Design review of the part built by this model. Coordinates are the model's own, in mm. A direction names the side the tool comes from. Round coordinates to 2 decimals unless told otherwise and drop trailing zeros. Write each loop counter-clockwise with the first axis right and the second up, starting at its lowest first coordinate (ties: lowest second). Pieces come first, ordered by that corner, then holes. Notation, with made-up numbers: (46, -26.5) - (85, -26.5) arc R9 cw to (85, -20.5) - close; hole circle Ø11 at (19, -24). An arc over 180 degrees is marked (long way). Use one line per item in the form item = value.
```python
from build123d import *

# Parameters (mm, degrees)
F1_DEPTH = 46.6
F2_W     = 38.3587293327
F2_H     = 9.7292885184
F3_DEPTH = 83.7873460183
F6_DEPTH = 23.8091403077


with BuildPart() as f1:
    # F0 (on Right) → F1 (new body, symmetric)
    with BuildSketch(Plane.YZ):
        Polygon((0, 19.4585770369), (0, 0), (83.7863460183, 0), (83.7863460183, 43.2667173445), align=None)
    extrude(amount=F1_DEPTH, both=True)

    # F2 (on face) → F3 (cut, through all)
    with BuildSketch(Plane.XZ):
        with Locations((0, 4.8646442592)):
            Rectangle(F2_W, F2_H)
    extrude(amount=-F3_DEPTH, mode=Mode.SUBTRACT)

    # F5 (on plane+point) → F6 (cut, through all)
    with BuildSketch(Plane.XY.offset(19.4585770369)):
        with BuildLine():
            Line((-19.1793646663, 0), (19.1793646663, 0))
            Line((19.1793646663, 0), (0.097478719, 83.3605036706))
            ThreePointArc((0.097478719, 83.3605036706), (0, 83.4381900123), (-0.097478719, 83.3605036706))
            Line((-0.097478719, 83.3605036706), (-19.1793646663, 0))
        make_face()
    extrude(amount=F6_DEPTH, mode=Mode.SUBTRACT)


solid = f1.part
```
Q1. We need section B-B on y = 35.5. Write out the cut boundary in (x, z), then the cut area to 3 significant figures.
Calculated:
outline = (-46.6, 0) - (-19.18, 0) - (-19.18, 9.73) - (19.18, 9.73) - (19.18, 0) - (46.6, 0) - (46.6, 29.55) - (11.05, 29.55) - (11.05, 19.46) - (-11.05, 19.46) - (-11.05, 29.55) - (-46.6, 29.55) - close
area = 2,160 mm2
Q2. We need section D-D on z = 34.5. Write out the cut boundary in (x, y), then the cut area to 3 significant figures.
Calculated:
outline = (-46.6, 52.93) - (-7.06, 52.93) - (-0.1, 83.36) arc R0.1 cw to (0.1, 83.36) - (7.06, 52.93) - (46.6, 52.93) - (46.6, 83.79) - (-46.6, 83.79) - close
area = 2,660 mm2
Q3. To check wall thickness, follow line 1 along X through (y, z) = (58.5, 2); line 2 along X through (y, z) = (42, 21.5); line 3 along Z through (x, y) = (3, 67). State the ranges of each line that lie inside material, in increasing order. Write a range as from..to.
Calculated:
line_1 = -46.6..-19.18, 19.18..46.6
line_2 = -46.6..-9.57, 9.57..46.6
line_3 = 9.73..19.46
Q4. We need section C-C on x = -2. Write out the cut boundary in (y, z), then the cut area to 3 significant figures.
Calculated:
outline = (0, 9.73) - (83.79, 9.73) - (83.79, 43.27) - (75.05, 40.78) - (75.05, 19.46) - (0, 19.46) - close
area = 1,010 mm2
Q5. Machinability: for faces 4 (the flat face through (33, 41, 0)), 5 (the flat face through (5.53, 59.62, 25.87)), 6 (the flat face through (19.179, 41, 5)), which of the approach directions +Z, -Z, +X, -X, +Y, -Y give a long, thin tool a straight path to every point of the face, cutting with its end or side? Answer none if there is none.
Calculated:
face_4 = -Z, +X, -X, +Y, -Y
face_5 = +Z, -Y
face_6 = -Z, +Y, -Y
Q6. For P1, Ø8, axis at x = 9.5, y = 66, coming from the -Z side; P2, Ø10, axis at x = 18.5, y = 63.5, coming from the +Z side; P3, Ø1.5, axis at x = -4.5, y = 62, coming from the +Z side, all flat-tipped, find the tip position at first contact; note any pin that passes through.
Calculated:
P1 = 9.73
P2 = 38.92
P3 = 37.27
Q7. Draft analysis for pull direction X (two halves, no side actions). For faces 1 (the flat face through (0, 33, 19.459)), 2 (the flat face through (1, 0, 10)), 3 (the flat face through (-46.6, 51, 17)), state which applies: released by +X, released by -X, zero draft, split by the parting line, or undercut.
Calculated:
face_1 = undercut
face_2 = zero draft
face_3 = released by -X
Q8. We need section A-A on z = 4. Write out the cut boundary in (x, y), then the cut area to 3 significant figures.
Calculated:
outline = (-46.6, 0) - (-19.18, 0) - (-19.18, 83.79) - (-46.6, 83.79) - close; (19.18, 0) - (46.6, 0) - (46.6, 83.79) - (19.18, 83.79) - close
area = 4,590 mm2
